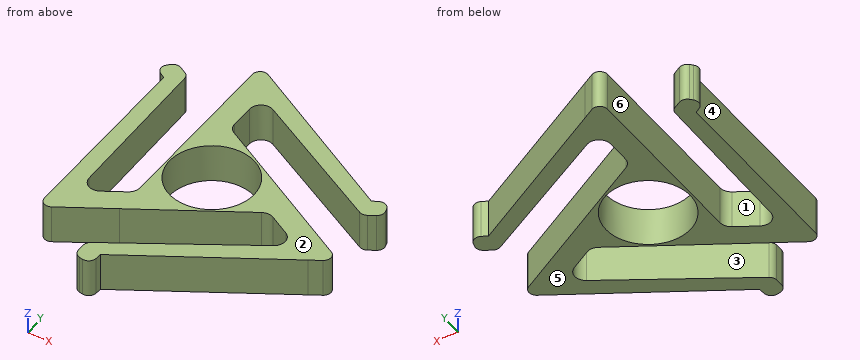
```python
from build123d import *

# Parameters (mm, degrees)
F0_R     = 11
F1_DEPTH = 10
F2_R     = 2
F3_R     = 3


with BuildPart() as f1:
    # F0 (on Top) → F1 (new body)
    with BuildSketch(Plane.XY):
        with BuildLine():
            Line((33.9994544901, 12.0421032112), (38.9284945409, 9.196320611))
            ThreePointArc((38.9284945409, 9.196320611), (38.3009590814, 11.5341464117), (37.5331647861, 13.8297339504))
            Line((37.5331647861, 13.8297339504), (33.9994544901, 12.0421032112))
        make_face()
        with BuildLine():
            Line((-27.4284945409, 23.4233396976), (-27.4284945409, 29.114904898))
            ThreePointArc((-27.4284945409, 29.114904898), (-29.1393433442, 27.4025303479), (-30.7434833217, 25.589807214))
            Line((-30.7434833217, 25.589807214), (-27.4284945409, 23.4233396976))
        make_face()
        with BuildLine():
            ThreePointArc((-11.5, -38.311225509), (-9.1616157371, -38.9366767596), (-6.7896814644, -39.4195411644))
            Line((-6.7896814644, -39.4195411644), (-6.5709599492, -35.4654429088))
            Line((-6.5709599492, -35.4654429088), (-11.5, -38.311225509))
        make_face()
        Polygon((-5.6430600129, 34.9297196308), (-11.5, 38.311225509), (-11.5, 32.768458128), (-5.6430600129, 29.496919338), align=None)
        Polygon((-27.4284945409, -22.3518931417), (-27.4284945409, -29.114904898), (-22.6283171817, -26.3435212075), (-22.7235514736, -19.6354929953), align=None)
        Polygon((33.0715545538, -12.5778264891), (38.9284945409, -9.196320611), (34.1283171817, -6.4249369205), (28.3666114865, -9.8614263427), align=None)
        Polygon((34.8825001806, 6.8603646779), (38.9284945409, 9.196320611), (33.9994544901, 12.0421032112), (-5.6430600129, 34.9297196308), (-5.6430600129, 29.496919338), align=None)
        Polygon((-23.3825001806, 26.778948965), (-27.4284945409, 29.114904898), (-27.4284945409, 23.4233396976), (-27.4284945409, -22.3518931417), (-22.7235514736, -19.6354929953), align=None)
        Polygon((-6.5709599492, -35.4654429088), (33.0715545538, -12.5778264891), (28.3666114865, -9.8614263427), (-11.5, -33.6393136429), (-11.5, -38.311225509), align=None)
        Polygon((17.1430600129, -3.3815058782), (23, 0), (-5.6430600129, 16.5370784089), (-11.5, 19.918584287), (-11.5, -13.1555725307), (-11.5, -19.918584287), align=None)
        Circle(F0_R, mode=Mode.SUBTRACT)
        Polygon((-5.6430600129, 16.5370784089), (-5.6430600129, 29.496919338), (-11.5, 32.768458128), (-11.5, 19.918584287), align=None)
        Polygon((-22.6283171817, -26.3435212075), (-11.5, -19.918584287), (-11.5, -13.1555725307), (-22.7235514736, -19.6354929953), align=None)
        Polygon((28.3666114865, -9.8614263427), (34.1283171817, -6.4249369205), (23, 0), (17.1430600129, -3.3815058782), align=None)
    extrude(amount=F1_DEPTH)

    # F2
    f2_edges = [f1.edges().sort_by_distance(p)[0] for p in [
        (37.533165, 13.829734, 5),
        (-11.5, 38.311226, 5),
        (38.928495, -9.196321, 5),
        (38.928495, 9.196321, 5),
        (34.8825, 6.860365, 5),
        (-6.789681, -39.419541, 5),
        (-11.5, -33.639314, 5),
        (-11.5, -38.311226, 5),
        (-27.428495, -29.114905, 5),
        (-30.743483, 25.589807, 5),
        (-27.428495, 29.114905, 5),
        (-23.3825, 26.778949, 5),
    ]]
    fillet(f2_edges, radius=F2_R)

    # F3
    f3_edges = [f1.edges().sort_by_distance(p)[0] for p in [
        (28.366611, -9.861426, 5),
        (17.14306, -3.381506, 5),
        (-5.64306, 16.537078, 5),
        (-5.64306, 29.496919, 5),
        (-11.5, -13.155573, 5),
        (-22.723551, -19.635493, 5),
    ]]
    fillet(f3_edges, radius=F3_R)


solid = f1.part
```
Input: part model. Units: mm. Frame: model coordinates. Face numbers are marked on the shaded views. A direction names the side the tool comes from. Round coordinates to 2 decimals unless told otherwise and drop trailing zeros. Loops run counter-clockwise (first coordinate to the right, second up) from the corner with the lowest first, then second, coordinate; pieces in that order, holes last. Notation, with made-up numbers: (12, -28.5) -> (58, -28.5) arc R29 cw to (58, 4.5) -> close; hole circle Ø4 at (44.25, 75.5). An arc over 180 degrees is marked (long way). Use one line per item in the form item = value. Start each with the question number.
Item 1: Section query D-D on y = -6. Return the cut outline in (x, z).
Item 2: Contact query for flat-ended pins moving along their axis: pin 1 Ø6 at (x, z) = (8.5, 7) entering from -Y; pin 2 Ø5 at (x, z) = (25, 6.5) entering from -Y; pin 3 Ø6 at (x, z) = (12.5, 3) entering from -Y. Output: stop coordinate, or through.
Item 3: Material intervals for L1, parallel to X at y = -11.5, z = 4; L2, parallel to X at y = 21, z = 5; L3, parallel to X at y = -8.5, z = 1, sorted ascending. Write a range as from..to.
Item 4: Section query B-B on y = 5.5. Return the cut outline in (x, z).
Item 5: Mould query, pull axis X, two halves, no side actions, for the marked faces 4, 5 and 6. Classes: pulls with the +X half, pulls with the -X half, needs draft (parallel to the pull), parting line crosses it, or undercut.
Item 6: Section query A-A on x = 20. Return the cut outline in (y, z), then the cut area to 3 significant figures.
Item 7: Set-up query: the marked faces 1, 2 and 3. Return all of +Z, -Z, +X, -X, +Y, -Y with unobstructed straight access to the full face (end or side cutting, diameter ignored); none if empty.
Item 8: Section query C-C on x = 0. Return the cut outline in (y, z).
Ans:
q1.outline = (-27.43, 0) -> (-22.92, 0) -> (-22.92, 10) -> (-27.43, 10) -> close; (-11.5, 0) -> (-9.22, 0) -> (-9.22, 10) -> (-11.5, 10) -> close; (9.22, 0) -> (12.61, 0) -> (12.61, 10) -> (9.22, 10) -> close; (21.68, 0) -> (33.39, 0) -> (33.39, 10) -> (21.68, 10) -> close
q2.pin_1 = -28.5
q2.pin_2 = -18.68
q2.pin_3 = -26.19
q3.L1 = -27.43..-22.84, -11.5..3.08, 24.98..34.94
q3.L2 = -27.43..-23.3, -11.5..-5.64, 9.57..18.48
q3.L3 = -27.43..-22.88, -11.5..-6.98, 6.98..8.28, 25.09..36.8
q4.outline = (-27.43, 0) -> (-23.08, 0) -> (-23.08, 10) -> (-27.43, 10) -> close; (-11.5, 0) -> (-9.53, 0) -> (-9.53, 10) -> (-11.5, 10) -> close; (9.53, 0) -> (13.47, 0) -> (13.47, 10) -> (9.53, 10) -> close
q5.face_4 = pulls with the -X half
q5.face_5 = needs draft
q5.face_6 = undercut
q6.outline = (-20.12, 0) -> (-14.85, 0) -> (-14.85, 10) -> (-20.12, 10) -> close; (-5.03, 0) -> (1.73, 0) -> (1.73, 10) -> (-5.03, 10) -> close; (15.17, 0) -> (20.12, 0) -> (20.12, 10) -> (15.17, 10) -> close
q6.area = 170 mm^2
q7.face_1 = +Z, -Z, +Y
q7.face_2 = +Z, +X, -X, +Y, -Y
q7.face_3 = +Z, -Z
q8.outline = (-31.67, 0) -> (-26.78, 0) -> (-26.78, 10) -> (-31.67, 10) -> close; (-13.28, 0) -> (-11, 0) -> (-11, 10) -> (-13.28, 10) -> close; (11, 0) -> (13.28, 0) -> (13.28, 10) -> (11, 10) -> close; (26.34, 0) -> (31.67, 0) -> (31.67, 10) -> (26.34, 10) -> close
